The model under review builds one solid part; all positions refer to its coordinate system, in mm. A direction names the side the tool comes from. Coordinates: 2 decimals unless noted, no trailing zeros. Order: outer loops, then holes, each group sorted by start corner. A loop starts at its lowest first (then second) coordinate and runs counter-clockwise, first axis right, second up. Notation, with made-up numbers: M -6,81.25 L 39,81.25 A10 cw 39,92.25 Z; hole C -27,29 d5. An arc over 180 degrees is marked long. One line per item, written item: value.
```python
from build123d import *

# Parameters (mm, degrees)
CUNA_DEPTH                        = 50
RECORTE_CARAS_PIRAMIDE_DEPTH      = 140.283882772
RECORTE_CARAS_PIRAMIDE_DEPTH_BACK = 140.283882772
CROQUIS_AGUJEROS_MONTAJE_R        = 4
AGUJERO_INSERTO_M6_DEPTH          = 14


with BuildPart() as part:
    # Croquis_triangulo_frontal → Cuna (new, symmetric)
    with BuildSketch(Plane.XY):
        Polygon((-50, 0), (50, 0), (0, 120), align=None)
    extrude(amount=CUNA_DEPTH, both=True)

    # Croquis_recorte_lateral → Recorte_caras_piramide (cut, two sides: drawn at the far end of the back side and taken through both)
    with BuildSketch(Plane(origin=(0, 0, 0), x_dir=(0, 0, -1), z_dir=(1, 0, 0)).offset(-RECORTE_CARAS_PIRAMIDE_DEPTH_BACK)):
        Polygon((-60, 0), (-50, 0), (0, 120), (50, 0), (60, 0), (60, 130), (-60, 130), align=None)
    extrude(amount=RECORTE_CARAS_PIRAMIDE_DEPTH + RECORTE_CARAS_PIRAMIDE_DEPTH_BACK, mode=Mode.SUBTRACT)

    # Croquis_agujeros_montaje → Agujero_inserto_M6 (cut)
    with BuildSketch(Plane(origin=(0, 0, 0), x_dir=(1, 0, 0), z_dir=(0, 1, 0))):
        with Locations(Location((0, 0, 0), (0, 0, 270))):
            Circle(CROQUIS_AGUJEROS_MONTAJE_R)
    extrude(amount=AGUJERO_INSERTO_M6_DEPTH, mode=Mode.SUBTRACT)


solid = part.part
```
(1) Insertion check: pin 1 Ø3 at (x, z) = (29, -34.5) entering from +Y; pin 2 Ø10 at (y, z) = (30, 29) entering from -X; pin 3 Ø10 at (x, y) = (0.5, 54) entering from -Z. Each pin has a flat end and moves straight along its axis. Give the tip position at first contact, or say it passes through.
Geometry results:
pin 1: stops at y = 40.8
pin 2: stops at x = -39.58
pin 3: stops at z = -29.58
(2) Mouldability with a two-part tool opening along X and no side actions: class faces 1 (the flat face through (30.906, 45.827, 0.7)), 2 (the flat face through (0, 14, 0)), 3 (the flat face through (-0.7, 45.827, 30.906)) as +X half, -X half, draft (parallel to the pull), parting line (faces both ways), or undercut.
Geometry results:
face 1: +X half
face 2: undercut
face 3: draft
(3) For L1, parallel to X at y = 9.25, z = 0; L2, parallel to X at y = 4.25, z = 0; L3, parallel to Y at x = -36, z = 15, list the stretches that pass through material, from the lowest coordinate up.
Geometry results:
L1: x = -46.15 to -4, 4 to 46.15
L2: x = -48.23 to -4, 4 to 48.23
L3: y = 0 to 33.6
(4) Tool access review of faces 4 (the flat face through (-1, 48, -30)), 5 (the cylindrical face through (-3.905, 6.902, -0.867)): name each direction out of +Z, -Z, +X, -X, +Y, -Y from which nothing blocks a thin tool from reaching the whole face with its end or side.
Geometry results:
face 4: -Z, +X, -X, +Y
face 5: -Y
(5) We need section B-B, the plane z = -10.5. State the section outline as (x, y) points.
Geometry results:
outline: M -50,0 L 50,0 L 10.5,94.8 L -10.5,94.8 Z
(6) We need section A-A, the plane x = -33. State the section outline as (y, z) points, plus the area to 3 significant figures.
Geometry results:
outline: M 0,-50 L 40.8,-33 L 40.8,33 L 0,50 Z
area: 3,390 mm2
